Part print with two shaded views. Sizes in mm from the minimum x, y, z corner. A direction names the side the tool comes from. Give positions to 0.01 mm unless a question says otherwise; leave off trailing zeros. Write each loop counter-clockwise with the first axis right and the second up, starting at its lowest first coordinate (ties: lowest second). Pieces come first, ordered by that corner, then holes. Notation, with made-up numbers: (43, 1.25) -> (89, 1.25) arc R25 cw to (89, 19.25) -> close; hole circle Ø4 at (-6, 31.5). An arc over 180 degrees is marked (long way). Write item = value, one per line. Start each with the question number.
Q1. Saw through at A-A, the plane y = 9.7. List the corners of the cut face in (x, z).
Q2. Drop flat-ended pins along their axis: P1, Ø3, axis at x = 13.94, y = 17.2, coming from the +Z side; P2, Ø1, axis at y = 4.5, z = 2.5, coming from the -X side; P3, Ø1.5, axis at y = 12, z = 2, coming from the -X side; P4, Ø2, axis at x = 26, z = 4, coming from the +Y side. Give the stop position or say it passes through.
Q3. Mould opens along Y. For the marked faces 4, 5, 6 and 7 say: pulls with the +Y half, pulls with the -Y half, needs draft (parallel to the pull), parting line crosses it, or undercut.
Q4. Tool access for the marked faces 1, 2 and 3: list every direction of +Z, -Z, +X, -X, +Y, -Y with a clear straight run to the whole face (end or side of a thin tool).
Q5. Saw through at B-B, the plane x = 25. List the corners of the cut face in (y, z).
Q6. Saw through at C-C, the plane z = 1.5. List the corners of the cut face in (x, y), then the cut area to 3 significant figures.
Q7. Wall check: line 1 (X direction, y = 9.7, z = 4.4); line 2 (Y direction, x = 24, z = 2.75); line 3 (Y direction, x = 10.25, z = 1.25). Give the ranges that are in metal, low to high.
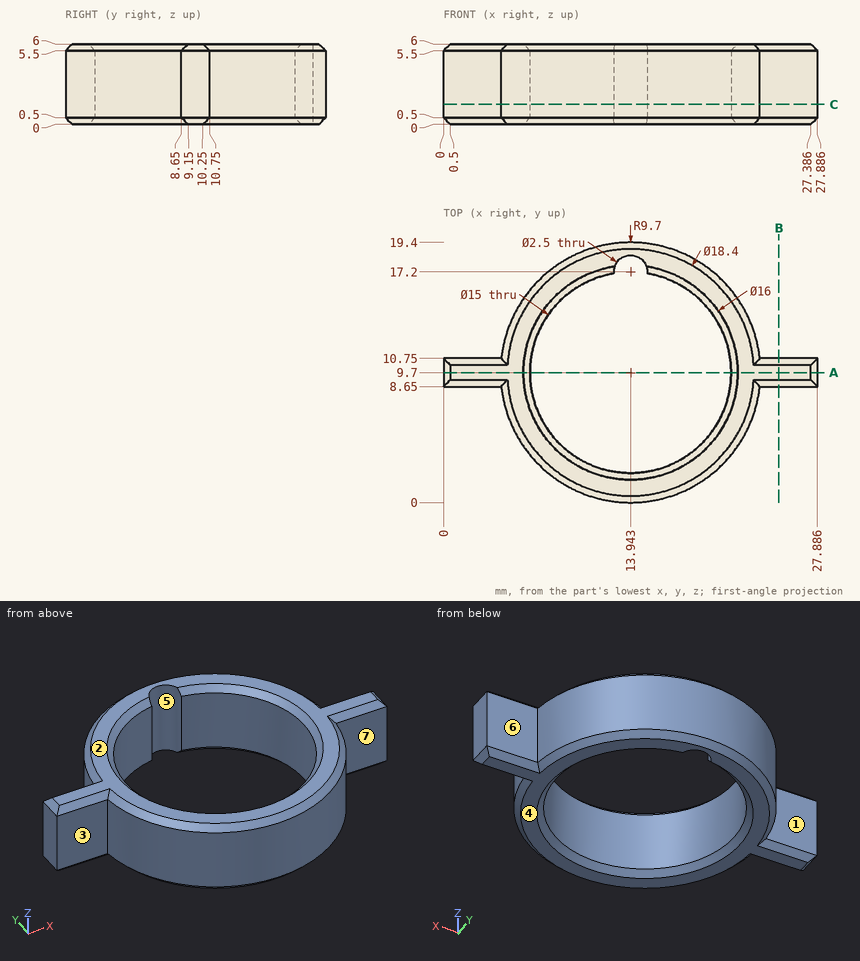
Report:
q1.outline = (0, 0.5) -> (0.5, 0) -> (5.94, 0) -> (6.44, 0.5) -> (6.44, 5.5) -> (5.94, 6) -> (0.5, 6) -> (0, 5.5) -> close; (21.44, 0.5) -> (21.94, 0) -> (27.39, 0) -> (27.89, 0.5) -> (27.89, 5.5) -> (27.39, 6) -> (21.94, 6) -> (21.44, 5.5) -> close
q2.P1 = 6
q2.P2 = 5.46
q2.P3 = 4.37
q2.P4 = 10.75
q3.face_4 = needs draft
q3.face_5 = undercut
q3.face_6 = pulls with the +Y half
q3.face_7 = pulls with the -Y half
q4.face_1 = +Z, -Z, -X, +Y
q4.face_2 = +Z, +X, -X, +Y, -Y
q4.face_3 = +Z, -Z, -X, -Y
q5.outline = (8.65, 0.5) -> (9.15, 0) -> (10.25, 0) -> (10.75, 0.5) -> (10.75, 5.5) -> (10.25, 6) -> (9.15, 6) -> (8.65, 5.5) -> close
q6.outline = (0, 8.65) -> (4.3, 8.65) arc R9.7 ccw to (23.59, 8.65) -> (27.89, 8.65) -> (27.89, 10.75) -> (23.59, 10.75) arc R9.7 ccw to (4.3, 10.75) -> (0, 10.75) -> close; hole (12.7, 17.1) arc R7.5 ccw (long way) to (15.19, 17.1) arc R1.25 ccw (long way) to start
q6.area = 134 mm2
q7.line_1 = 0 to 6.44, 21.44 to 27.89
q7.line_2 = 8.65 to 10.75
q7.line_3 = 0.73 to 3.17, 16.23 to 18.67
